Model file for the job. Use its own axes, mm. Face numbers are marked on the shaded views. A direction names the side the tool comes from. Coordinates: 2 decimals unless noted, no trailing zeros. Order: outer loops, then holes, each group sorted by start corner. A loop starts at its lowest first (then second) coordinate and runs counter-clockwise, first axis right, second up.
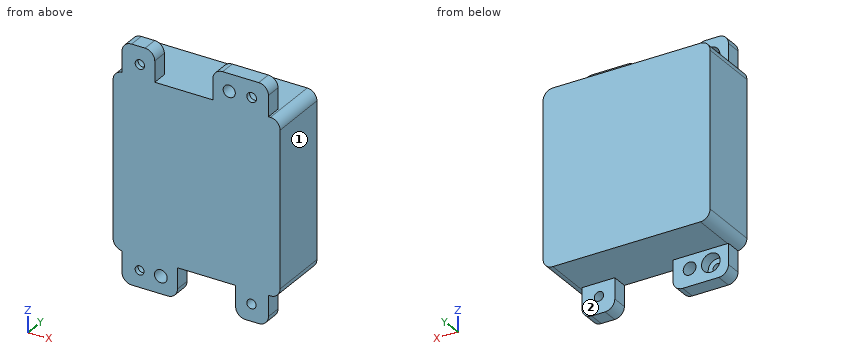
from build123d import *

# Parameters (mm, degrees)
SKETCH1_W                  = 27.2796
SKETCH1_H                  = 28.5242
ENCLOSURE_DEPTH            = 9.7536
SKETCH2_W                  = 9.0678
SKETCH2_H                  = 4.9784
SKETCH2_W_2                = 5.3594
MOUNTING_TABS_DEPTH        = 2.54
SMALL_MOUNTING_HOLES_REACH = 26.663
SKETCH3_R                  = 1.0414
SKETCH3_R_2                = 0.9906
LARGE_MOUNTING_HOLES_REACH = 27.522
SKETCH4_R                  = 0.762
SKETCH4_R_2                = 0.7874
SKETCH4_R_3                = 0.7239
SKETCH5_R                  = 1.524
CUT_EXTRUDE1_DEPTH         = 1.778
FILLET1_R                  = 1.5875
FILLET2_R                  = 1.5875


with BuildPart() as part:
    # Sketch1 → Enclosure (new body)
    with BuildSketch(Plane(origin=(0, 0, 0), x_dir=(1, 0, 0), z_dir=(0, 1, 0))):
        Rectangle(SKETCH1_W, SKETCH1_H)
    extrude(amount=ENCLOSURE_DEPTH)

    # Sketch2 → Mounting Tabs (add)
    with BuildSketch(Plane(origin=(0, 0, 0), x_dir=(1, 0, 0), z_dir=(0, 1, 0))):
        with Locations((-7.6581, 16.7513)):
            Rectangle(SKETCH2_W, SKETCH2_H)
        with Locations((9.0551, 16.7513)):
            Rectangle(SKETCH2_W_2, SKETCH2_H)
        with Locations((-9.5123, -16.7513)):
            Rectangle(SKETCH2_W_2, SKETCH2_H)
        with Locations((7.2009, -16.7513)):
            Rectangle(SKETCH2_W, SKETCH2_H)
    extrude(amount=MOUNTING_TABS_DEPTH)

    # Sketch3 → Small Mounting Holes (cut, up to next)
    with BuildSketch(Plane(origin=(0, 2.54, 0), x_dir=(1, 0, 0), z_dir=(0, 1, 0)), mode=Mode.PRIVATE) as small_mounting_holes_sk1:
        with Locations(Location((-5.842, 16.4211, 0), (0, 0, 270))):
            Circle(SKETCH3_R)
    small_mounting_holes_tool1 = extrude(small_mounting_holes_sk1.sketch, amount=-SMALL_MOUNTING_HOLES_REACH, mode=Mode.PRIVATE) & part.part
    # Sketch3 → Small Mounting Holes (cut, up to next)
    with BuildSketch(Plane(origin=(0, 2.54, 0), x_dir=(1, 0, 0), z_dir=(0, 1, 0)), mode=Mode.PRIVATE) as small_mounting_holes_sk2:
        with Locations(Location((5.334, -16.4211, 0), (0, 0, 270))):
            Circle(SKETCH3_R_2)
    small_mounting_holes_tool2 = extrude(small_mounting_holes_sk2.sketch, amount=-SMALL_MOUNTING_HOLES_REACH, mode=Mode.PRIVATE) & part.part
    add(small_mounting_holes_tool1.solids().sort_by_distance((-5.842, 2.54, -16.4211))[0], mode=Mode.SUBTRACT)
    add(small_mounting_holes_tool2.solids().sort_by_distance((5.334, 2.54, 16.4211))[0], mode=Mode.SUBTRACT)

    # Sketch4 → Large Mounting Holes (cut, up to next)
    with BuildSketch(Plane.XZ, mode=Mode.PRIVATE) as large_mounting_holes_sk1:
        with Locations(Location((-9.271, 16.3703, 0), (0, 0, 270))):
            Circle(SKETCH4_R)
    large_mounting_holes_tool1 = extrude(large_mounting_holes_sk1.sketch, amount=-LARGE_MOUNTING_HOLES_REACH, mode=Mode.PRIVATE) & part.part
    # Sketch4 → Large Mounting Holes (cut, up to next)
    with BuildSketch(Plane.XZ, mode=Mode.PRIVATE) as large_mounting_holes_sk2:
        with Locations(Location((8.9916, 16.5227, 0), (0, 0, 270))):
            Circle(SKETCH4_R_2)
    large_mounting_holes_tool2 = extrude(large_mounting_holes_sk2.sketch, amount=-LARGE_MOUNTING_HOLES_REACH, mode=Mode.PRIVATE) & part.part
    # Sketch4 → Large Mounting Holes (cut, up to next)
    with BuildSketch(Plane.XZ, mode=Mode.PRIVATE) as large_mounting_holes_sk3:
        with Locations(Location((8.9662, -16.4719, 0), (0, 0, 270))):
            Circle(SKETCH4_R)
    large_mounting_holes_tool3 = extrude(large_mounting_holes_sk3.sketch, amount=-LARGE_MOUNTING_HOLES_REACH, mode=Mode.PRIVATE) & part.part
    # Sketch4 → Large Mounting Holes (cut, up to next)
    with BuildSketch(Plane.XZ, mode=Mode.PRIVATE) as large_mounting_holes_sk4:
        with Locations(Location((-9.3091, -16.51, 0), (0, 0, 270))):
            Circle(SKETCH4_R_3)
    large_mounting_holes_tool4 = extrude(large_mounting_holes_sk4.sketch, amount=-LARGE_MOUNTING_HOLES_REACH, mode=Mode.PRIVATE) & part.part
    add(large_mounting_holes_tool1.solids().sort_by_distance((-9.271, 0, 16.3703))[0], mode=Mode.SUBTRACT)
    add(large_mounting_holes_tool2.solids().sort_by_distance((8.9916, 0, 16.5227))[0], mode=Mode.SUBTRACT)
    add(large_mounting_holes_tool3.solids().sort_by_distance((8.9662, 0, -16.4719))[0], mode=Mode.SUBTRACT)
    add(large_mounting_holes_tool4.solids().sort_by_distance((-9.3091, 0, -16.51))[0], mode=Mode.SUBTRACT)

    # Sketch5 → Cut-Extrude1 (cut)
    with BuildSketch(Plane(origin=(0, 2.54, 0), x_dir=(1, 0, 0), z_dir=(0, 1, 0))):
        with Locations(Location((-9.271, -16.3703, 0), (0, 0, 270))):
            Circle(SKETCH5_R)
        with Locations(Location((8.9916, -16.5227, 0), (0, 0, 270))):
            Circle(SKETCH5_R)
        with Locations(Location((-9.3091, 16.51, 0), (0, 0, 270))):
            Circle(SKETCH5_R)
    extrude(amount=-CUT_EXTRUDE1_DEPTH, mode=Mode.SUBTRACT)

    # Fillet1
    fillet1_edges = [part.edges().sort_by_distance(p)[0] for p in [
        (-13.6398, 4.8768, -14.2621),
        (13.6398, 4.8768, -14.2621),
        (-13.6398, 4.8768, 14.2621),
        (13.6398, 4.8768, 14.2621),
    ]]
    fillet(fillet1_edges, radius=FILLET1_R)

    # Fillet2
    fillet2_edges = [part.edges().sort_by_distance(p)[0] for p in [
        (-12.192, 1.27, 19.2405),
        (2.667, 1.27, 19.2405),
        (-6.8326, 1.27, 19.2405),
        (11.7348, 1.27, 19.2405),
        (-12.192, 1.27, -19.2405),
        (-3.1242, 1.27, -19.2405),
        (6.3754, 1.27, -19.2405),
        (11.7348, 1.27, -19.2405),
    ]]
    fillet(fillet2_edges, radius=FILLET2_R)


solid = part.part
Q1. Which spindle directions (+Z, -Z, +X, -X, +Y, -Y) get a long thin tool onto all of the face, cutting with end or side? Do the marked faces 1 and 2. Say none if no direction does.
Established:
face 1: +Z, -Z, +X, +Y, -Y
face 2: -Z, +X, -X, +Y
Q2. Cut at A-A, the plane y = 5. List the corners of the cut face in (x, z) (1 decimal), plus the area to 3 significant figures.
Established:
outline: (-13.6, -12.7) arc R1.6 ccw to (-12.1, -14.3) - (12.1, -14.3) arc R1.6 ccw to (13.6, -12.7) - (13.6, 12.7) arc R1.6 ccw to (12.1, 14.3) - (-12.1, 14.3) arc R1.6 ccw to (-13.6, 12.7) - close
area: 776 mm2
Q3. Cut at D-D, the plane y = 1.75. Count the separate pieces of the cut face and the enclosed holes in it, plus the area to 3 significant figures.
Established:
separate pieces: 1
enclosed holes: 6
area: 885 mm2
Q4. Cut at B-B, the plane z = -16.51. List the corners of the cut face in (x, y), plus the area to 3 significant figures.
Established:
outline: (-12.19, 0) - (-10.03, 0) - (-10.03, 0.76) - (-10.83, 0.76) - (-10.83, 2.54) - (-12.19, 2.54) - close; (-8.59, 0) - (-6.88, 0) - (-6.88, 2.54) - (-7.79, 2.54) - (-7.79, 0.76) - (-8.59, 0.76) - close; (-4.8, 0) - (-3.12, 0) - (-3.12, 2.54) - (-4.8, 2.54) - close; (6.38, 0) - (8.21, 0) - (8.21, 2.54) - (6.38, 2.54) - close; (9.73, 0) - (11.73, 0) - (11.73, 2.54) - (9.73, 2.54) - close
area: 21.0 mm2
Q5. Probe line 1 (X direction, y = 0.2, z = -16.51); line 2 (Z direction, x = 10.5, y = 3.5); line 3 (Z direction, x = -5.25, y = 2). List the from-to ranges inside material, lowest first.
Established:
line 1: x = -12.19 to -10.03, -8.59 to -6.88, -4.8 to -3.12, 6.38 to 8.21, 9.73 to 11.73
line 2: z = -14.26 to 14.26
line 3: z = -19.24 to -17.28, -15.56 to 14.26
Q6. Cut at C-C, the plane x = -2. List the corners of the cut face in (y, z), plus the area to 3 significant figures.
Established:
outline: (0, -14.26) - (9.75, -14.26) - (9.75, 14.26) - (0, 14.26) - close
area: 278 mm2
Q7. Drop flat-ended pins along their axis: P1, Ø2.5, axis at x = 9.5, z = -17, coming from the +Y side; P2, Ø3, axis at y = 8.5, z = 13, coming from the +X side; P3, Ø3, axis at x = 0, y = 5, coming from the +Z side; P4, Ø1.7, axis at x = -5.84, z = -16.42, coming from the +Y side. Give the stop position or say it passes through.
Established:
P1: stops at y = 2.54
P2: stops at x = 13.64
P3: stops at z = 14.26
P4: passes through
